Could you check a few things on this model? Use its own coordinates, in mm. A direction names the side the tool comes from. Give positions to 0.01 mm unless a question says otherwise; leave off trailing zeros. Order: outer loops, then holes, each group sorted by start corner. A loop starts at its lowest first (then second) coordinate and runs counter-clockwise, first axis right, second up.
(1) Imagine slicing it at B-B, the plane x = -58. Write out the boundary of the cut face in (y, z).
(2) Imagine slicing it at A-A, the plane y = -44. Write out the boundary of the cut face in (x, z).
(3) On a 3-axis mill with a long thin cutter (end or side, diameter ignored), from which of +Z, -Z, +X, -X, +Y, -Y can I reach the whole of each face in a straight line? I mean faces 1 (the flat face through (7.124, -24.14, 202.465)), 2 (the flat face through (-15, -12, 205)). Say none if no direction works.
(4) Imagine slicing it at C-C, the plane z = 136. Write out the boundary of the cut face in (x, y), then the cut area to 3 significant figures.
(5) Will these pins go through, and if not, where does the flat tip stop? pin 1 (5 mm diameter, centred on y = -25.5, z = 83, fed in from +X); pin 2 (10 mm diameter, centred on y = 45.5, z = 41.5, fed in from +X); pin 3 (12 mm diameter, centred on y = -16.5, z = -34.5, fed in from -X).
(6) If I drill on probe 1 along Y at (x, z) = (-15.5, -30); probe 2 along Y at (x, z) = (-11, 60.5); probe 3 along X at (y, z) = (62.5, 6), over which ranges is the centre line in solid material (lowest first)?
(7) If we mould it in two halves opening along X, with no side actions, what happens to faces 3 (the flat face through (-6, 2, -100)), 4 (the flat face through (12.97, -23.68, 74.82)), 5 (the cylindrical face through (-17.902, 9.387, 202.465)), 6 (the flat face through (26.406, -19.137, 117.082))? For each: released by +X, released by -X, zero draft, split by the parting line, or undercut.
(8) Imagine slicing it at D-D, the plane x = 55. Write out the boundary of the cut face in (y, z).
from build123d import *

# Parameters (mm, degrees)
F16_R     = 7.9698515936
F16_R_2   = 7.9172343221
F17_DEPTH = 5


with BuildPart() as f3:
    # F0 (on Top) → F3 section 0
    with BuildSketch(Plane.XY, mode=Mode.PRIVATE) as f3_s0:
        Polygon((0.4073861914, 72.1302863076), (-62.6703534203, -35.7123363628), (62.2629672289, -36.4179499447), align=None)
    loft([f3_s0.sketch, Vertex(0, 0, 100)])

    # F4 (on offset) → F5 section 0
    with BuildSketch(Plane.XY.offset(100), mode=Mode.PRIVATE) as f5_s0:
        Polygon((72.1279709711, 0.706893576), (-36.6761732802, 62.1112083964), (-35.4517976909, -62.8181019724), align=None)
    loft([f5_s0.sketch, Vertex(0, 0, 0)])

    # F5_face (on face) → F10 section 0
    with BuildSketch(Plane.XY.offset(100), mode=Mode.PRIVATE) as f10_s0:
        Polygon((-35.4517976909, -62.8181019724), (72.1279709711, 0.706893576), (-36.6761732802, 62.1112083964), align=None)
    loft([f10_s0.sketch, Vertex(0, 0, 200)])

    # F3_face (on face) → F11 section 0
    with BuildSketch(Plane(origin=(0, 0, 0), x_dir=(1, 0, 0), z_dir=(0, 0, -1)), mode=Mode.PRIVATE) as f11_s0:
        Polygon((-62.6703534203, 35.7123363628), (0.4073861914, -72.1302863076), (62.2629672289, 36.4179499447), align=None)
    loft([f11_s0.sketch, Vertex(0, 0, -100)])

    # F12 (on offset) → F13 section 0
    with BuildSketch(Plane.XY.offset(200), mode=Mode.PRIVATE) as f13_s0:
        Polygon((-72.1151262546, 1.5337731971), (34.729276575, -63.2204179321), (37.3858496796, 61.686644735), align=None)
    loft([f13_s0.sketch, Vertex(0, 0, 0)])

    # F14 (on offset) → F15 section 0
    with BuildSketch(Plane.XY.offset(-100), mode=Mode.PRIVATE) as f15_s0:
        Polygon((3.9172189187, -72.0249907385), (60.4168622275, 39.404906465), (-64.3340811462, 32.6200842734), align=None)
    loft([f15_s0.sketch, Vertex(0, 0, 0)])

    # F16 (on offset) → F17 (join)
    with BuildSketch(Plane.XY.offset(200)):
        with Locations((-14.4072528929, -12.0968222618)):
            Circle(F16_R)
        with Locations((-11.618857272, 14.2046045512)):
            Circle(F16_R_2)
        with BuildLine():
            Line((0, -20.3613266349), (14.4505379722, -28.0257780105))
            add(Edge.make_bspline(
                [(14.4505379722, -28.0257780105), (20.5031350206, -19.362007973), (32.2544355779, -2.5410359414), (14.4116547637, 23.9984281751), (13.5612826949, 24.6133738576), (13.4361311793, 24.7038770467)],
                knots=[0, 0, 0, 0, 0.4752828108, 0.9227759779, 1, 1, 1, 1], degree=3))
            Line((13.4361311793, 24.7038770467), (0, 24.1440590471))
            add(Edge.make_bspline(
                [(0, -20.3613266349), (7.3122692601, -12.4437830296), (21.681873302, 3.1152674575), (7.141301884, 17.2178609781), (0, 24.1440590471)],
                knots=[0, 0, 0, 0, 0.508870616, 1, 1, 1, 1], degree=3))
        make_face()
    extrude(amount=F17_DEPTH)


solid = f3.part
Answer block:
1. outline: (-35.74, 0) - (-33.05, -7.45) - (-27.73, 0) - (-33.05, 7.45) - close; (-7.02, 200) - (1.23, 160.85) - (9.29, 200) - close; (22.91, -100) - (32.96, -100) - (29.41, -90.15) - close
2. outline: (-35.64, 100) - (-24.83, 70.04) - (-3.58, 100) - (-24.83, 129.96) - close; (-14.36, -100) - (18.13, -100) - (2.39, -61.09) - close; (3.02, 200) - (24.17, 139.2) - (35.14, 200) - close
3. face 1: +Z, -X, -Y
3. face 2: +Z, +X, -X, +Y, -Y
4. outline: (-49.04, 1.04) - (-22.94, -14.78) - (-22.69, -40.2) - (-1.56, -27.73) - (23.62, -42.99) - (24.26, -12.48) - (46.16, 0.45) - (24.8, 12.51) - (25.42, 41.95) - (-1.33, 27.25) - (-23.47, 39.75) - (-23.23, 15.22) - close
4. area: 3,940 mm2
5. pin 1: stops at x = 20.28
5. pin 2: stops at x = 1.88
5. pin 3: stops at x = -41.33
6. probe 1: y = -25.16 to 23.5
6. probe 2: y = -31.84 to 31.26
6. probe 3: x = -2.72 to 3.4
7. face 3: zero draft
7. face 4: released by +X
7. face 5: undercut
7. face 6: undercut
8. outline: (-36.38, 0) - (-32.17, -11.66) - (-23.67, 0) - (-32.17, 11.66) - close; (-9.41, 100) - (0.54, 76.25) - (10.37, 100) - (0.54, 123.75) - close; (28.72, -100) - (39.11, -100) - (35.87, -91.03) - close
